```python
from build123d import *

# Parameters (mm, degrees)
SKETCH1_W               = 121.57
SKETCH1_H               = 61
BOSS_EXTRUDE1_DEPTH     = 3.235369433
SKETCH2_W               = 121.57
SKETCH2_H               = 61
SKETCH2_W_2             = 115.57
SKETCH2_H_2             = 55
BOSS_EXTRUDE2_DEPTH     = 37
CUT_EXTRUDE1_REACH      = 123.57
SKETCH3_W               = 14.3
SKETCH3_H               = 11.7
SKETCH5_W               = 2
SKETCH5_H               = 55
BOSS_EXTRUDE3_DEPTH     = 35
SKETCH7_R               = 5
CUT_EXTRUDE3_DEPTH      = 20
CHAMFER10_SIZE          = 2
SKETCH8_R               = 0.75
CUT_EXTRUDE4_DEPTH      = 11
CUT_EXTRUDE4_DEPTH_BACK = 17


with BuildPart() as part:
    # Sketch1 → Boss-Extrude1 (new body)
    with BuildSketch(Plane(origin=(0, 0, 0), x_dir=(1, 0, 0), z_dir=(0, 1, 0))):
        Rectangle(SKETCH1_W, SKETCH1_H)
    extrude(amount=BOSS_EXTRUDE1_DEPTH)

    # Sketch2 → Boss-Extrude2 (add)
    with BuildSketch(Plane(origin=(0, 3.235369433, 0), x_dir=(1, 0, 0), z_dir=(0, 1, 0))):
        Rectangle(SKETCH2_W, SKETCH2_H)
        Rectangle(SKETCH2_W_2, SKETCH2_H_2, mode=Mode.SUBTRACT)
    extrude(amount=BOSS_EXTRUDE2_DEPTH)

    # Sketch3 → Cut-Extrude1 (cut, up to next)
    with BuildSketch(Plane.ZY.offset(60.785), mode=Mode.PRIVATE) as cut_extrude1_sk1:
        with Locations((-11.35, 20.35)):
            Rectangle(SKETCH3_W, SKETCH3_H)
    cut_extrude1_tool1 = extrude(cut_extrude1_sk1.sketch, amount=-CUT_EXTRUDE1_REACH, mode=Mode.PRIVATE) & part.part
    add(cut_extrude1_tool1.solids().sort_by_distance((-60.785, 20.35, -11.35))[0], mode=Mode.SUBTRACT)

    # Sketch5 → Boss-Extrude3 (add)
    with BuildSketch(Plane(origin=(0, 3.235369433, 0), x_dir=(1, 0, 0), z_dir=(0, 1, 0))):
        with Locations((17.93, 0)):
            Rectangle(SKETCH5_W, SKETCH5_H)
    extrude(amount=BOSS_EXTRUDE3_DEPTH)

    # Sketch7 → Cut-Extrude3 (cut)
    with BuildSketch(Plane.XY.offset(30.5)):
        with Locations((40.785, 21.15)):
            Circle(SKETCH7_R)
    extrude(amount=-CUT_EXTRUDE3_DEPTH, mode=Mode.SUBTRACT)

    # Chamfer10
    chamfer10_edges = [part.edges().sort_by_distance(p)[0] for p in [
        (35.785, 21.15, 30.5),
    ]]
    chamfer(chamfer10_edges, length=CHAMFER10_SIZE)

    # Sketch8 → Cut-Extrude4 (cut, two sides)
    with BuildSketch(Plane.ZY.offset(-16.93)) as cut_extrude4_sk:
        with Locations((-0.737087906, 12.579188257)):
            Circle(SKETCH8_R)
        with Locations((1.278476701, 12.579188257)):
            Circle(SKETCH8_R)
        with Locations((3.44541986, 12.579188257)):
            Circle(SKETCH8_R)
        with Locations((5.769363075, 12.579188257)):
            Circle(SKETCH8_R)
        with Locations((-2.774299402, 12.579188257)):
            Circle(SKETCH8_R)
    extrude(amount=CUT_EXTRUDE4_DEPTH, mode=Mode.SUBTRACT)
    extrude(cut_extrude4_sk.sketch, amount=-CUT_EXTRUDE4_DEPTH_BACK, mode=Mode.SUBTRACT)


solid = part.part
```
Here's how the part is built. I have some questions about the finished solid (model axes, mm). A direction names the side the tool comes from. Give positions to 0.01 mm unless a question says otherwise; leave off trailing zeros. Write each loop counter-clockwise with the first axis right and the second up, starting at its lowest first coordinate (ties: lowest second). Pieces come first, ordered by that corner, then holes. Notation, with made-up numbers: (15.25, 20.5) -> (61.25, 20.5) arc R22 cw to (61.25, 39.5) -> close; hole circle Ø11 at (32.5, 37.25). An arc over 180 degrees is marked (long way). Use one line per item in the form item = value.
1) Suppose I cut it at C-C (z = 19.5). Please give me the cut outline in (x, y) (3 decimals), and give its area (3 significant figures).
Verdict:
outline = (-60.785, 0) -> (60.785, 0) -> (60.785, 40.235) -> (57.785, 40.235) -> (57.785, 3.235) -> (18.93, 3.235) -> (18.93, 38.235) -> (16.93, 38.235) -> (16.93, 3.235) -> (-57.785, 3.235) -> (-57.785, 40.235) -> (-60.785, 40.235) -> close
area = 685 mm2
2) We'd pull the mould along Z, two halves only. Please class faces 5 (the face through (16.93, 20, 0)), 6 (the face through (-1, 20, -30.5)), 7 (the face through (-1, 20, 30.5)), 8 (the face through (-1, 0, 0)): +Z half, -Z half, draft (parallel to the pull), parting line (faces both ways), or undercut.
Verdict:
face_5 = undercut
face_6 = -Z half
face_7 = +Z half
face_8 = draft
3) If I drill on L1, parallel to X at y = 14, z = 2.5 (3 decimals); L2, parallel to Z at x = -19, y = 38.5; L3, parallel to X at y = 21, z = 28 (3 decimals), over which ranges is the centre line in solid material (lowest first)? Write a range as [from, to].
Verdict:
L1 = [-60.785, -57.785], [16.93, 18.93], [57.785, 60.785]
L2 = [-30.5, -27.5], [27.5, 30.5]
L3 = [-60.785, 35.787], [45.783, 60.785]
4) Suppose I cut it at B-B (x = 25.5). Please give me the cut outline in (y, z).
Verdict:
outline = (0, -30.5) -> (40.24, -30.5) -> (40.24, -27.5) -> (3.24, -27.5) -> (3.24, 27.5) -> (40.24, 27.5) -> (40.24, 30.5) -> (0, 30.5) -> close
5) On a 3-axis mill with a long thin cutter (end or side, diameter ignored), from which of +Z, -Z, +X, -X, +Y, -Y can I reach the whole of each face in a straight line? I mean faces 1 (the face through (57.785, 21, 0)), 2 (the face through (-59, 20, -4.2)), 3 (the face through (60.785, 20, 0)), 4 (the face through (37.1, 24.53, 28.01)). Say none if no direction works.
Verdict:
face_1 = +Y
face_2 = -X
face_3 = +Z, -Z, +X, +Y, -Y
face_4 = +Z
6) Suppose I cut it at D-D (y = 21.15). Please give me the cut outline in (x, z) (3 decimals), and give its area (3 significant figures).
Verdict:
outline = (-60.785, -30.5) -> (60.785, -30.5) -> (60.785, 30.5) -> (47.785, 30.5) -> (45.785, 28.5) -> (45.785, 27.5) -> (57.785, 27.5) -> (57.785, -27.5) -> (18.93, -27.5) -> (18.93, 27.5) -> (35.785, 27.5) -> (35.785, 28.5) -> (33.785, 30.5) -> (-60.785, 30.5) -> (-60.785, -4.2) -> (-57.785, -4.2) -> (-57.785, 27.5) -> (16.93, 27.5) -> (16.93, -27.5) -> (-57.785, -27.5) -> (-57.785, -18.5) -> (-60.785, -18.5) -> close
area = 1,090 mm2
7) Suppose I cut it at A-A (y = 36). Please give me the cut outline in (x, z) (3 decimals), and give its area (3 significant figures).
Verdict:
outline = (-60.785, -30.5) -> (60.785, -30.5) -> (60.785, 30.5) -> (-60.785, 30.5) -> close; hole (-57.785, -27.5) -> (16.93, -27.5) -> (16.93, 27.5) -> (-57.785, 27.5) -> close; hole (18.93, -27.5) -> (57.785, -27.5) -> (57.785, 27.5) -> (18.93, 27.5) -> close
area = 1,170 mm2
8) I'm going to push flat-ended pins straight in: pin 1 (1 mm diameter, centred on x = 16.5, z = -9, fed in from +Y); pin 2 (16.5 mm diameter, centred on x = -13.5, z = 8.5, fed in from +Y); pin 3 (3 mm diameter, centred on x = 27, z = 12.5, fed in from -Y); pin 4 (8 mm diameter, centred on y = 19.5, z = -13.5, fed in from -X). Where does each tip first touch, or does it pass through?
Verdict:
pin_1 = 38.24
pin_2 = 3.24
pin_3 = 0
pin_4 = 16.93
